Could you check a few things on this model? Use its own coordinates, in mm. A direction names the side the tool comes from. Coordinates: 2 decimals unless noted, no trailing zeros. Write each loop counter-clockwise with the first axis right and the second up, starting at its lowest first coordinate (ties: lowest second). Pieces come first, ordered by that corner, then holes. Notation, with made-up numbers: (22, -25) - (51, -25) arc R29 cw to (51, 11) - close; hole circle Ø5 at (53.5, 16.5). An arc over 180 degrees is marked (long way). Write item = value, one per line. Start each with the question number.
```python
from build123d import *

# Parameters (mm, degrees)
F0_R     = 15.875
F1_DEPTH = 31.75
F2_R     = 6.35
F3_DEPTH = 76.2
F4_R     = 4.1275
F5_DEPTH = 76.2


with BuildPart() as f1:
    # F0 (on Top) → F1 (new body)
    with BuildSketch(Plane.XY):
        Circle(F0_R)
    extrude(amount=-F1_DEPTH)

    # F2 (on Top) → F3 (join)
    with BuildSketch(Plane.XY):
        Circle(F2_R)
    extrude(amount=-F3_DEPTH)

    # F4 (on Right) → F5 (join, symmetric)
    with BuildSketch(Plane.YZ):
        with Locations((0, -15.875)):
            Circle(F4_R)
    extrude(amount=F5_DEPTH, both=True)


solid = f1.part
```
1) Suppose I cut it at C-C on z = -8.5. Please give me the cut outline in (x, y) (3 decimals).
2) Which directions (+Z, -Z, +X, -X, +Y, -Y) give clear straight access to the entire face, cutting with the end or side of a thin tool? Please do faces 1 (the flat face through (7, 0, -31.75)), 2 (the cylindrical face through (-45.338, 2.219, -12.395)), 3 (the flat face through (0, 0, 0)), 4 (the cylindrical face through (46.191, 2.219, -12.395)), 5 (the flat face through (-76.2, 0, -16)).
3) Suppose I cut it at D-D on x = -25. Please give me the cut outline in (y, z) (1 decimal).
4) For P1, Ø4, axis at x = 54.5, y = -4, coming from the -Z side; P2, Ø10, axis at x = -51, y = 0.5, coming from the +Z side; P3, Ø3, axis at y = -3, z = -53.5, coming from the -X side, each with a flat end and sliding along its axis, tell me the tip position at first contact or that it passes through.
5) Suppose I cut it at A-A on x = 0. Please give me the cut outline in (y, z) (3 decimals), plus the area to 3 significant figures.
6) If I drill on probe 1 along Z at (x, y) = (4, -10); probe 2 along X at (y, z) = (6, -22); probe 3 along Z at (x, y) = (-50, -2), over which ranges is the centre line in solid material (lowest first)? Write a range as [from, to].
Reply:
q1.outline = circle Ø31.75 at (0, 0)
q2.face_1 = -Z
q2.face_2 = -X
q2.face_3 = +Z, +X, -X, +Y, -Y
q2.face_4 = +X
q2.face_5 = +Z, -Z, -X, +Y, -Y
q3.outline = circle Ø8.3 at (0, -15.9)
q4.P1 = -19.49
q4.P2 = -11.75
q4.P3 = -6.17
q5.outline = (-15.875, -31.75) - (-6.35, -31.75) - (-6.35, -76.2) - (6.35, -76.2) - (6.35, -31.75) - (15.875, -31.75) - (15.875, 0) - (-15.875, 0) - close
q5.area = 1,570 mm^2
q6.probe_1 = [-31.75, 0]
q6.probe_2 = [-14.7, 14.7]
q6.probe_3 = [-19.49, -12.26]
